For this review, take the finished solid that the model builds, in its own axes (mm). A direction names the side the tool comes from. Give positions to 0.01 mm unless a question says otherwise; leave off trailing zeros. Write each loop counter-clockwise with the first axis right and the second up, starting at its lowest first coordinate (ties: lowest second). Pieces come first, ordered by that corner, then holes.
1) We need section A-A on x = 6. Give the boundary of the cut face in (y, z), and give its area (3 significant figures).
2) Draft analysis for pull direction Y (two halves, no side actions). For faces 3 (the face through (-1, -16.574, -451)), 4 (the face through (0, -20.638, -451)), 5 (the face through (17, -1, 0)), state which applies: pulls with the +Y half, pulls with the -Y half, needs draft (parallel to the pull), parting line crosses it, or undercut.
3) Machinability: for faces 1 (the face through (16.574, 0, -451)), 2 (the face through (20.638, 0, -451)), which of the approach directions +Z, -Z, +X, -X, +Y, -Y give a long, thin tool a straight path to every point of the face, cutting with its end or side? Answer none if there is none.
4) For P1, Ø1.2, axis at x = 19, z = -326, coming from the -Y side; P2, Ø2, axis at y = 6, z = -351, coming from the -X side; P3, Ø2, axis at x = 19.5, z = -789.5, coming from the +Y side, all flat-tipped, find the tip position at first contact; note any pin that passes through.
5) Wall thickness on line 1 along X through (y, z) = (15.5, -423); line 2 along Y through (x, z) = (-9.5, -367); line 3 along Y through (x, z) = (-18, -75) (1 decimal): over which ranges is each line inside the solid? List them lowest first.
from build123d import *

# Parameters (mm, degrees)
EXTRUDE_THIN1_DEPTH = 914.4
FILLET2_R           = 0.762
FILLET3_R           = 1.524
CUT_EXTRUDE1_DEPTH  = 916.563701788
LPATTERN1_COUNT     = 18
LPATTERN1_PITCH     = 50.8


with BuildPart() as part:
    # Sketch1 → Extrude-Thin1 (new body)
    with BuildSketch(Plane.XY):
        with BuildLine():
            Line((-13.5255, 9.525), (-18.2499, 9.525))
            ThreePointArc((-18.2499, 9.525), (-19.938188151, 10.224311849), (-20.6375, 11.9126))
            Line((-20.6375, 11.9126), (-20.6375, 18.2499))
            ThreePointArc((-20.6375, 18.2499), (-19.938188151, 19.938188151), (-18.2499, 20.6375))
            Line((-18.2499, 20.6375), (18.2499, 20.6375))
            ThreePointArc((18.2499, 20.6375), (19.938188151, 19.938188151), (20.6375, 18.2499))
            Line((20.6375, 18.2499), (20.6375, -18.2499))
            ThreePointArc((20.6375, -18.2499), (19.938188151, -19.938188151), (18.2499, -20.6375))
            Line((18.2499, -20.6375), (-18.2499, -20.6375))
            ThreePointArc((-18.2499, -20.6375), (-19.938188151, -19.938188151), (-20.6375, -18.2499))
            Line((-20.6375, -18.2499), (-20.6375, -11.9126))
            ThreePointArc((-20.6375, -11.9126), (-19.938188151, -10.224311849), (-18.2499, -9.525))
            Line((-18.2499, -9.525), (-13.5255, -9.525))
            Line((-13.5255, -9.525), (-13.5255, -13.589))
            Line((-13.5255, -13.589), (-16.5735, -13.589))
            Line((-16.5735, -13.589), (-16.5735, -16.5735))
            Line((-16.5735, -16.5735), (16.5735, -16.5735))
            Line((16.5735, -16.5735), (16.5735, 16.5735))
            Line((16.5735, 16.5735), (-16.5735, 16.5735))
            Line((-16.5735, 16.5735), (-16.5735, 13.589))
            Line((-16.5735, 13.589), (-13.5255, 13.589))
            Line((-13.5255, 13.589), (-13.5255, 9.525))
        make_face()
    extrude(amount=-EXTRUDE_THIN1_DEPTH)

    # Fillet2
    fillet2_edges = [part.edges().sort_by_distance(p)[0] for p in [
        (-16.5735, -13.589, -457.2),
        (-16.5735, -16.5735, -457.2),
        (-16.5735, 16.5735, -457.2),
        (-16.5735, 13.589, -457.2),
        (-13.5255, 13.589, -457.2),
        (-13.5255, 9.525, -457.2),
        (-13.5255, -9.525, -457.2),
        (-13.5255, -13.589, -457.2),
    ]]
    fillet(fillet2_edges, radius=FILLET2_R)

    # Fillet3
    fillet3_edges = [part.edges().sort_by_distance(p)[0] for p in [
        (16.5735, -16.5735, -457.2),
        (16.5735, 16.5735, -457.2),
    ]]
    fillet(fillet3_edges, radius=FILLET3_R)

    # Sketch2 → Cut-Extrude1 (cut, through all)
    with BuildSketch(Plane(origin=(20.6375, 0, 0), x_dir=(0, 0, -1), z_dir=(1, 0, 0))):
        with BuildLine():
            Line((15.875, 4.7625), (31.75, 4.7625))
            ThreePointArc((31.75, 4.7625), (36.5125, 0), (31.75, -4.7625))
            Line((31.75, -4.7625), (15.875, -4.7625))
            ThreePointArc((15.875, -4.7625), (11.1125, 0), (15.875, 4.7625))
        make_face()
    cut_extrude1 = extrude(amount=-CUT_EXTRUDE1_DEPTH, mode=Mode.SUBTRACT)

    # LPattern1: Cut-Extrude1 ×18
    with Locations(*[(0, 0, -i * LPATTERN1_PITCH) for i in range(1, LPATTERN1_COUNT)]):
        add(cut_extrude1, mode=Mode.SUBTRACT)


solid = part.part
Results list:
1. outline: (-20.64, -914.4) - (-16.57, -914.4) - (-16.57, 0) - (-20.64, 0) - close; (16.57, -914.4) - (20.64, -914.4) - (20.64, 0) - (16.57, 0) - close
1. area: 7,430 mm2
2. face 3: undercut
2. face 4: pulls with the -Y half
2. face 5: needs draft
3. face 1: +Z, -Z
3. face 2: +Z, -Z, +X, +Y, -Y
4. P1: stops at y = -20.63
4. P2: stops at x = 16.57
4. P3: stops at y = 20.62
5. line 1: x = -20.64 to -16.57, 16.51 to 20.64
5. line 2: y = -20.64 to -16.57, 16.57 to 20.64
5. line 3: y = -20.6 to -9.5, 9.5 to 20.6
